Could you check a few things on this model? Use its own coordinates, in mm. Face numbers are marked on the shaded views. Give positions to 0.01 mm unless a question says otherwise; leave off trailing zeros. Loops run counter-clockwise (first coordinate to the right, second up) from the corner with the lowest first, then second, coordinate; pieces in that order, holes last.
1. For P1, Ø4.5, axis at y = -3.5, z = 0.5, coming from the +X side; P2, Ø1.2, axis at x = 0.5, y = -4.5, coming from the +Z side; P3, Ø10, axis at x = 13.5, z = -33, coming from the -Y side, each with a flat end and sliding along its axis, tell me the tip position at first contact or that it passes through.
2. Imagine slicing it at C-C (y = 2.25). List the corners of the cut face in (x, z) for me, plus the area to 3 significant figures.
3. Imagine slicing it at A-A (x = -39). List the corners of the cut face in (y, z) for me.
4. Imagine slicing it at B-B (z = -19.5). List the corners of the cut face in (x, y) for me, plus the area to 3 significant figures.
5. Thinking about a two-plate mould opening in Z: for the marked faces 1 and 2, which applies, +Z half, -Z half, draft (parallel to the pull), parting line (faces both ways), or undercut?
6. I need wall thicknesses on line 1 along X through (y, z) = (2.75, 36); line 2 along Z through (x, y) = (-82, 2.5); line 3 along Y through (x, z) = (26, -28.5). Which ranges of each line are inside material? Lowest first, please.
7. Imagine slicing it at D-D (z = -6.5). List the corners of the cut face in (x, y) for me, plus the area to 3 significant figures.
```python
from build123d import *

# Parameters (mm, degrees)
SKETCH1_W           = 53.5
SKETCH1_H           = 77
BOSS_EXTRUDE1_DEPTH = 4
SKETCH2_W           = 40
SKETCH2_H           = 20
BOSS_EXTRUDE2_DEPTH = 2
SKETCH3_W           = 40
SKETCH3_H           = 20
BOSS_EXTRUDE3_DEPTH = 4


with BuildPart() as part:
    # Sketch1 → Boss-Extrude1 (new body)
    with BuildSketch(Plane(origin=(0, 0, 0), x_dir=(1, 0, 0), z_dir=(0, 1, 0))):
        with BuildLine():
            Line((-87.5, 42.5), (87.5, 42.5))
            Line((87.5, 42.5), (90.5, 35.7))
            Line((90.5, 35.7), (90.5, -40.5))
            ThreePointArc((90.5, -40.5), (89.035533906, -44.035533906), (85.5, -45.5))
            Line((85.5, -45.5), (-85.5, -45.5))
            ThreePointArc((-85.5, -45.5), (-89.035533906, -44.035533906), (-90.5, -40.5))
            Line((-90.5, -40.5), (-90.5, 35.7))
            Line((-90.5, 35.7), (-87.5, 42.5))
        make_face()
        with Locations((-56.75, 0)):
            Rectangle(SKETCH1_W, SKETCH1_H, mode=Mode.SUBTRACT)
    extrude(amount=BOSS_EXTRUDE1_DEPTH)

    # Sketch2 → Boss-Extrude2 (add)
    with BuildSketch(Plane(origin=(0, 0, 0), x_dir=(1, 0, 0), z_dir=(0, 1, 0))):
        Rectangle(SKETCH2_W, SKETCH2_H)
    extrude(amount=-BOSS_EXTRUDE2_DEPTH)

    # Sketch3 → Boss-Extrude3 (add)
    # profile 1 of 5: a face of its own
    with BuildSketch(Plane(origin=(0, -2, 0), x_dir=(1, 0, 0), z_dir=(0, 1, 0))):
        Rectangle(SKETCH3_W, SKETCH3_H)
        Polygon((-2, 9), (0, 9), (2, 9), (17.5, 9), (17.5, 2), (17.5, 0), (17.5, -2), (17.5, -9), (2, -9), (0, -9), (-2, -9), (-17.5, -9), (-17.5, -2), (-17.5, 0), (-17.5, 2), (-17.5, 9), align=None, mode=Mode.SUBTRACT)
    # profile 2 of 5: a face of its own
    with BuildSketch(Plane(origin=(0, -2, 0), x_dir=(1, 0, 0), z_dir=(0, 1, 0))):
        Polygon((-17.5, 2), (-2, 9), (-17.5, 9), align=None)
    # profile 3 of 5: a face of its own
    with BuildSketch(Plane(origin=(0, -2, 0), x_dir=(1, 0, 0), z_dir=(0, 1, 0))):
        Polygon((-2, -9), (-17.5, -2), (-17.5, -9), align=None)
    # profile 4 of 5: a face of its own
    with BuildSketch(Plane(origin=(0, -2, 0), x_dir=(1, 0, 0), z_dir=(0, 1, 0))):
        Polygon((17.5, -9), (17.5, -2), (2, -9), align=None)
    # profile 5 of 5: a face of its own
    with BuildSketch(Plane(origin=(0, -2, 0), x_dir=(1, 0, 0), z_dir=(0, 1, 0))):
        Polygon((17.5, 9), (2, 9), (17.5, 2), align=None)
    extrude(amount=-BOSS_EXTRUDE3_DEPTH)


solid = part.part
```
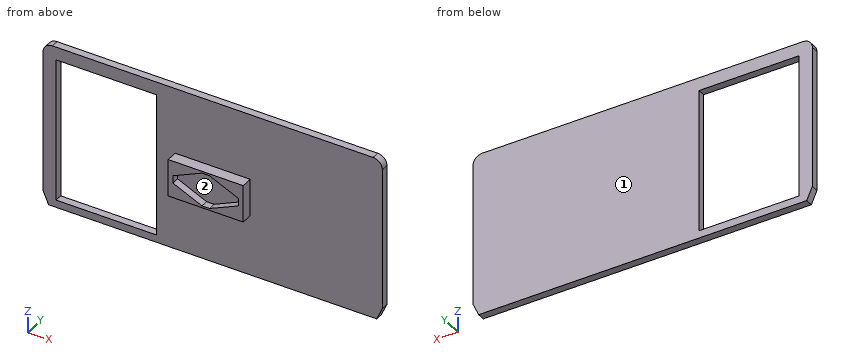
Derived:
1. P1: stops at x = 20
1. P2: stops at z = 10
1. P3: stops at y = 0
2. outline: (-90.5, -35.7) - (-87.5, -42.5) - (87.5, -42.5) - (90.5, -35.7) - (90.5, 40.5) arc R5 ccw to (85.5, 45.5) - (-85.5, 45.5) arc R5 ccw to (-90.5, 40.5) - close; hole (-83.5, -38.5) - (-30, -38.5) - (-30, 38.5) - (-83.5, 38.5) - close
2. area: 11,800 mm2
3. outline: (0, -42.5) - (4, -42.5) - (4, -38.5) - (0, -38.5) - close; (0, 38.5) - (4, 38.5) - (4, 45.5) - (0, 45.5) - close
4. outline: (-90.5, 0) - (-83.5, 0) - (-83.5, 4) - (-90.5, 4) - close; (-30, 0) - (90.5, 0) - (90.5, 4) - (-30, 4) - close
4. area: 510 mm2
5. face 1: draft
5. face 2: undercut
6. line 1: x = -90.5 to -83.5, -30 to 90.5
6. line 2: z = -42.5 to -38.5, 38.5 to 45.5
6. line 3: y = 0 to 4
7. outline: (-90.5, 0) - (-83.5, 0) - (-83.5, 4) - (-90.5, 4) - close; (-30, 0) - (-20, 0) - (-20, -6) - (-7.54, -6) - (-7.54, -2) - (7.54, -2) - (7.54, -6) - (20, -6) - (20, 0) - (90.5, 0) - (90.5, 4) - (-30, 4) - close
7. area: 690 mm2
